from build123d import *

# Parameters (mm, degrees)
F1_DEPTH = 25
F2_R     = 5
F3_R     = 4
F4_DEPTH = 47.8


with BuildPart() as f1:
    # F0 (on Front) → F1 (new body)
    with BuildSketch(Plane.XZ):
        with BuildLine():
            Line((-5, 5), (-5, 29.5803989155))
            ThreePointArc((-5, 29.5803989155), (-21.2132034356, 21.2132034356), (-29.5803989155, 5))
            Line((-29.5803989155, 5), (-5, 5))
        make_face()
    extrude(amount=F1_DEPTH)

    # F2
    f2_edges = [f1.edges().sort_by_distance(p)[0] for p in [
        (-5, -12.5, 5),
    ]]
    fillet(f2_edges, radius=F2_R)

    # F3 (on Front) → F4 (cut)
    with BuildSketch(Plane.XZ):
        with Locations((-15.5563491861, 15.5563491861)):
            Circle(F3_R)
    extrude(amount=F4_DEPTH, mode=Mode.SUBTRACT)


solid = f1.part
Input: part model. Units: mm. Frame: model coordinates. Coordinates: 2 decimals unless noted, no trailing zeros. Write each loop counter-clockwise with the first axis right and the second up, starting at its lowest first coordinate (ties: lowest second). Pieces come first, ordered by that corner, then holes. Notation, with made-up numbers: M 59,-19 L 100,-19 A12 cw 100,-6 Z; hole C 38.25,1 d9. An arc over 180 degrees is marked long. Answer as a JSON object with one key per item and string values. Group by question number.
(1) Contact query for flat-ended pins moving along their axis: P1, Ø3, axis at x = -13.5, y = -11, coming from the +Z side; P2, Ø3, axis at x = -13, y = -21, coming from the +Z side; P3, Ø4, axis at x = -12.5, y = -3.5, coming from the +Z side. Output: stop coordinate, or through.
(2) Mould query, pull axis X, two halves, no side actions, for faces 1 (the face through (-5, -12, 20)), 2 (the face through (-21.029, -12.325, 21.396)), 3 (the face through (-13.41, -12.32, 18.93)), 4 (the face through (-20, -12, 5)). Classes: pulls with the +X half, pulls with the -X half, needs draft (parallel to the pull), parting line crosses it, or undercut.
(3) Section A-A on x = -12. Output: boundary loops of the cut face in (y, z).
(4) Section B-B on z = 12. Output: boundary loops of the cut face in (x, y).
(5) Section C-C on y = -8.5. Output: boundary loops of the cut face in (x, z).
(6) Section D-D on z = 22. Output: boundary loops of the cut face in (x, y), plus the area to 3 significant figures.
(7) Ray query, line 1 along X through (y, z) = (-23, 22.75); line 2 along X through (y, z) = (-20.5, 13.75); line 3 along Z through (x, y) = (-14.5, -17.5). Return the intervals inside material, ascending. Write a range as [from, to].
Result set:
{
 "1": {"P1": "stops at z = 27.5", "P2": "stops at z = 27.71", "P3": "stops at z = 28.1"},
 "2": {"face 1": "pulls with the +X half", "face 2": "pulls with the -X half", "face 3": "undercut", "face 4": "needs draft"},
 "3": {"outline": "M -25,5 L 0,5 L 0,13.73 L -25,13.73 Z; M -25,17.39 L 0,17.39 L 0,27.5 L -25,27.5 Z"},
 "4": {"outline": "M -27.5,-25 L -17.39,-25 L -17.39,0 L -27.5,0 Z; M -13.73,-25 L -5,-25 L -5,0 L -13.73,0 Z"},
 "5": {"outline": "M -29.58,5 L -10,5 A5 ccw -5,10 L -5,29.58 A30 ccw Z; hole C -15.56,15.56 d8"},
 "6": {"outline": "M -20.4,-25 L -5,-25 L -5,0 L -20.4,0 Z", "area": "385 mm2"},
 "7": {"line 1": "x = [-19.56, -5]", "line 2": "x = [-26.66, -19.13], [-11.99, -5]", "line 3": "z = [5, 11.7], [19.41, 26.26]"}
}
